CAD build for the part. Positions are in the model's coordinates, mm. Give positions to 0.01 mm unless a question says otherwise; leave off trailing zeros. Order: outer loops, then holes, each group sorted by start corner. A loop starts at its lowest first (then second) coordinate and runs counter-clockwise, first axis right, second up. Notation, with made-up numbers: (-38.75, 18.5) -> (-18.75, 18.5) arc R24 ccw to (-18.75, 49.5) -> close; hole circle Ø1 at (0.5, 57). An arc over 180 degrees is marked (long way). Answer as CSV lines item,"result".
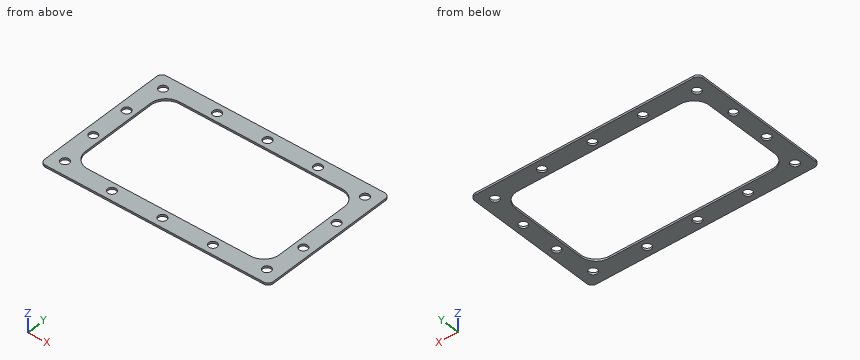
```python
from build123d import *

# Parameters (mm, degrees)
SKETCH1_W           = 112
SKETCH1_H           = 70
BOSS_EXTRUDE1_DEPTH = 1
FILLET1_R           = 3
SKETCH3_W           = 94
SKETCH3_H           = 52
CUT_EXTRUDE2_DEPTH  = 67.045438904
FILLET2_R           = 7.5
CUT_EXTRUDE3_REACH  = 68.045
SKETCH4_R           = 1.6
SKETCH5_R           = 2.05
CUT_EXTRUDE4_DEPTH  = 67.045438904
SKETCH6_W           = 132
SKETCH6_H           = 90
CUT_EXTRUDE5_DEPTH  = 67.045438904


with BuildPart() as part:
    # Sketch1 → Boss-Extrude1 (new body)
    with BuildSketch(Plane.XY):
        Rectangle(SKETCH1_W, SKETCH1_H)
    extrude(amount=BOSS_EXTRUDE1_DEPTH)

    # Fillet1
    fillet1_edges = [part.edges().sort_by_distance(p)[0] for p in [
        (-56, 35, 0.5),
        (56, 35, 0.5),
        (56, -35, 0.5),
        (-56, -35, 0.5),
    ]]
    fillet(fillet1_edges, radius=FILLET1_R)

    # Sketch3 → Cut-Extrude2 (cut, through all)
    with BuildSketch(Plane(origin=(0, 0, 0), x_dir=(-1, 0, 0), z_dir=(0, 0, -1))):
        Rectangle(SKETCH3_W, SKETCH3_H)
    extrude(amount=-CUT_EXTRUDE2_DEPTH, mode=Mode.SUBTRACT)

    # Fillet2
    fillet2_edges = [part.edges().sort_by_distance(p)[0] for p in [
        (-47, 26, 0.5),
        (-47, -26, 0.5),
        (47, -26, 0.5),
        (47, 26, 0.5),
    ]]
    fillet(fillet2_edges, radius=FILLET2_R)

    # Sketch4 → Cut-Extrude3 (cut, up to next)
    with BuildSketch(Plane(origin=(0, 0, 0), x_dir=(-1, 0, 0), z_dir=(0, 0, -1)), mode=Mode.PRIVATE) as cut_extrude3_sk1:
        with Locations((49, -28)):
            Circle(SKETCH4_R)
    cut_extrude3_tool1 = extrude(cut_extrude3_sk1.sketch, amount=-CUT_EXTRUDE3_REACH, mode=Mode.PRIVATE) & part.part
    # Sketch4 → Cut-Extrude3 (cut, up to next)
    with BuildSketch(Plane(origin=(0, 0, 0), x_dir=(-1, 0, 0), z_dir=(0, 0, -1)), mode=Mode.PRIVATE) as cut_extrude3_sk2:
        with Locations((24.5, -30)):
            Circle(SKETCH4_R)
    cut_extrude3_tool2 = extrude(cut_extrude3_sk2.sketch, amount=-CUT_EXTRUDE3_REACH, mode=Mode.PRIVATE) & part.part
    # Sketch4 → Cut-Extrude3 (cut, up to next)
    with BuildSketch(Plane(origin=(0, 0, 0), x_dir=(-1, 0, 0), z_dir=(0, 0, -1)), mode=Mode.PRIVATE) as cut_extrude3_sk3:
        with Locations((0, -30)):
            Circle(SKETCH4_R)
    cut_extrude3_tool3 = extrude(cut_extrude3_sk3.sketch, amount=-CUT_EXTRUDE3_REACH, mode=Mode.PRIVATE) & part.part
    # Sketch4 → Cut-Extrude3 (cut, up to next)
    with BuildSketch(Plane(origin=(0, 0, 0), x_dir=(-1, 0, 0), z_dir=(0, 0, -1)), mode=Mode.PRIVATE) as cut_extrude3_sk4:
        with Locations((-24.5, -30)):
            Circle(SKETCH4_R)
    cut_extrude3_tool4 = extrude(cut_extrude3_sk4.sketch, amount=-CUT_EXTRUDE3_REACH, mode=Mode.PRIVATE) & part.part
    # Sketch4 → Cut-Extrude3 (cut, up to next)
    with BuildSketch(Plane(origin=(0, 0, 0), x_dir=(-1, 0, 0), z_dir=(0, 0, -1)), mode=Mode.PRIVATE) as cut_extrude3_sk5:
        with Locations((-49, -28)):
            Circle(SKETCH4_R)
    cut_extrude3_tool5 = extrude(cut_extrude3_sk5.sketch, amount=-CUT_EXTRUDE3_REACH, mode=Mode.PRIVATE) & part.part
    # Sketch4 → Cut-Extrude3 (cut, up to next)
    with BuildSketch(Plane(origin=(0, 0, 0), x_dir=(-1, 0, 0), z_dir=(0, 0, -1)), mode=Mode.PRIVATE) as cut_extrude3_sk6:
        with Locations((-51, -9.5)):
            Circle(SKETCH4_R)
    cut_extrude3_tool6 = extrude(cut_extrude3_sk6.sketch, amount=-CUT_EXTRUDE3_REACH, mode=Mode.PRIVATE) & part.part
    # Sketch4 → Cut-Extrude3 (cut, up to next)
    with BuildSketch(Plane(origin=(0, 0, 0), x_dir=(-1, 0, 0), z_dir=(0, 0, -1)), mode=Mode.PRIVATE) as cut_extrude3_sk7:
        with Locations((-51, 9.5)):
            Circle(SKETCH4_R)
    cut_extrude3_tool7 = extrude(cut_extrude3_sk7.sketch, amount=-CUT_EXTRUDE3_REACH, mode=Mode.PRIVATE) & part.part
    # Sketch4 → Cut-Extrude3 (cut, up to next)
    with BuildSketch(Plane(origin=(0, 0, 0), x_dir=(-1, 0, 0), z_dir=(0, 0, -1)), mode=Mode.PRIVATE) as cut_extrude3_sk8:
        with Locations((-49, 28)):
            Circle(SKETCH4_R)
    cut_extrude3_tool8 = extrude(cut_extrude3_sk8.sketch, amount=-CUT_EXTRUDE3_REACH, mode=Mode.PRIVATE) & part.part
    # Sketch4 → Cut-Extrude3 (cut, up to next)
    with BuildSketch(Plane(origin=(0, 0, 0), x_dir=(-1, 0, 0), z_dir=(0, 0, -1)), mode=Mode.PRIVATE) as cut_extrude3_sk9:
        with Locations((-24.5, 30)):
            Circle(SKETCH4_R)
    cut_extrude3_tool9 = extrude(cut_extrude3_sk9.sketch, amount=-CUT_EXTRUDE3_REACH, mode=Mode.PRIVATE) & part.part
    # Sketch4 → Cut-Extrude3 (cut, up to next)
    with BuildSketch(Plane(origin=(0, 0, 0), x_dir=(-1, 0, 0), z_dir=(0, 0, -1)), mode=Mode.PRIVATE) as cut_extrude3_sk10:
        with Locations((0, 30)):
            Circle(SKETCH4_R)
    cut_extrude3_tool10 = extrude(cut_extrude3_sk10.sketch, amount=-CUT_EXTRUDE3_REACH, mode=Mode.PRIVATE) & part.part
    # Sketch4 → Cut-Extrude3 (cut, up to next)
    with BuildSketch(Plane(origin=(0, 0, 0), x_dir=(-1, 0, 0), z_dir=(0, 0, -1)), mode=Mode.PRIVATE) as cut_extrude3_sk11:
        with Locations((24.5, 30)):
            Circle(SKETCH4_R)
    cut_extrude3_tool11 = extrude(cut_extrude3_sk11.sketch, amount=-CUT_EXTRUDE3_REACH, mode=Mode.PRIVATE) & part.part
    # Sketch4 → Cut-Extrude3 (cut, up to next)
    with BuildSketch(Plane(origin=(0, 0, 0), x_dir=(-1, 0, 0), z_dir=(0, 0, -1)), mode=Mode.PRIVATE) as cut_extrude3_sk12:
        with Locations((49, 28)):
            Circle(SKETCH4_R)
    cut_extrude3_tool12 = extrude(cut_extrude3_sk12.sketch, amount=-CUT_EXTRUDE3_REACH, mode=Mode.PRIVATE) & part.part
    # Sketch4 → Cut-Extrude3 (cut, up to next)
    with BuildSketch(Plane(origin=(0, 0, 0), x_dir=(-1, 0, 0), z_dir=(0, 0, -1)), mode=Mode.PRIVATE) as cut_extrude3_sk13:
        with Locations((51, 9.5)):
            Circle(SKETCH4_R)
    cut_extrude3_tool13 = extrude(cut_extrude3_sk13.sketch, amount=-CUT_EXTRUDE3_REACH, mode=Mode.PRIVATE) & part.part
    # Sketch4 → Cut-Extrude3 (cut, up to next)
    with BuildSketch(Plane(origin=(0, 0, 0), x_dir=(-1, 0, 0), z_dir=(0, 0, -1)), mode=Mode.PRIVATE) as cut_extrude3_sk14:
        with Locations((51, -9.5)):
            Circle(SKETCH4_R)
    cut_extrude3_tool14 = extrude(cut_extrude3_sk14.sketch, amount=-CUT_EXTRUDE3_REACH, mode=Mode.PRIVATE) & part.part
    add(cut_extrude3_tool1.solids().sort_by_distance((-49, -28, 0))[0], mode=Mode.SUBTRACT)
    add(cut_extrude3_tool2.solids().sort_by_distance((-24.5, -30, 0))[0], mode=Mode.SUBTRACT)
    add(cut_extrude3_tool3.solids().sort_by_distance((0, -30, 0))[0], mode=Mode.SUBTRACT)
    add(cut_extrude3_tool4.solids().sort_by_distance((24.5, -30, 0))[0], mode=Mode.SUBTRACT)
    add(cut_extrude3_tool5.solids().sort_by_distance((49, -28, 0))[0], mode=Mode.SUBTRACT)
    add(cut_extrude3_tool6.solids().sort_by_distance((51, -9.5, 0))[0], mode=Mode.SUBTRACT)
    add(cut_extrude3_tool7.solids().sort_by_distance((51, 9.5, 0))[0], mode=Mode.SUBTRACT)
    add(cut_extrude3_tool8.solids().sort_by_distance((49, 28, 0))[0], mode=Mode.SUBTRACT)
    add(cut_extrude3_tool9.solids().sort_by_distance((24.5, 30, 0))[0], mode=Mode.SUBTRACT)
    add(cut_extrude3_tool10.solids().sort_by_distance((0, 30, 0))[0], mode=Mode.SUBTRACT)
    add(cut_extrude3_tool11.solids().sort_by_distance((-24.5, 30, 0))[0], mode=Mode.SUBTRACT)
    add(cut_extrude3_tool12.solids().sort_by_distance((-49, 28, 0))[0], mode=Mode.SUBTRACT)
    add(cut_extrude3_tool13.solids().sort_by_distance((-51, 9.5, 0))[0], mode=Mode.SUBTRACT)
    add(cut_extrude3_tool14.solids().sort_by_distance((-51, -9.5, 0))[0], mode=Mode.SUBTRACT)

    # Sketch5 → Cut-Extrude4 (cut, through all)
    with BuildSketch(Plane.XY.offset(1)):
        with Locations((-49, 28)):
            Circle(SKETCH5_R)
        with Locations((-24.5, 30)):
            Circle(SKETCH5_R)
        with Locations((0, 30)):
            Circle(SKETCH5_R)
        with Locations((24.5, 30)):
            Circle(SKETCH5_R)
        with Locations((49, 28)):
            Circle(SKETCH5_R)
        with Locations((51, 9.5)):
            Circle(SKETCH5_R)
        with Locations((51, -9.5)):
            Circle(SKETCH5_R)
        with Locations((49, -28)):
            Circle(SKETCH5_R)
        with Locations((24.5, -30)):
            Circle(SKETCH5_R)
        with Locations((0, -30)):
            Circle(SKETCH5_R)
        with Locations((-24.5, -30)):
            Circle(SKETCH5_R)
        with Locations((-49, -28)):
            Circle(SKETCH5_R)
        with Locations((-51, -9.5)):
            Circle(SKETCH5_R)
        with Locations((-51, 9.5)):
            Circle(SKETCH5_R)
    extrude(amount=-CUT_EXTRUDE4_DEPTH, mode=Mode.SUBTRACT)

    # Sketch6 → Cut-Extrude5 (cut, through all)
    with BuildSketch(Plane.XY.offset(1)):
        Rectangle(SKETCH6_W, SKETCH6_H)
        with BuildLine():
            Line((-53, 34.5), (53, 34.5))
            ThreePointArc((53, 34.5), (54.767766953, 33.767766953), (55.5, 32))
            Line((55.5, 32), (55.5, -32))
            ThreePointArc((55.5, -32), (54.767766953, -33.767766953), (53, -34.5))
            Line((53, -34.5), (-53, -34.5))
            ThreePointArc((-53, -34.5), (-54.767766953, -33.767766953), (-55.5, -32))
            Line((-55.5, -32), (-55.5, 32))
            ThreePointArc((-55.5, 32), (-54.767766953, 33.767766953), (-53, 34.5))
        make_face(mode=Mode.SUBTRACT)
    extrude(amount=-CUT_EXTRUDE5_DEPTH, mode=Mode.SUBTRACT)


solid = part.part
```
1) Wall check: line 1 along Y through (x, z) = (-24.5, 0.4); line 2 along Y through (x, z) = (40.5, 0.15); line 3 along Y through (x, z) = (7.5, 0.3). Give the ranges that are in metal, low to high. Write a range as [from, to].
Data:
line 1,"y = [-34.5, -32.05], [-27.95, -26], [26, 27.95], [32.05, 34.5]"
line 2,"y = [-34.5, -25.93], [25.93, 34.5]"
line 3,"y = [-34.5, -26], [26, 34.5]"
2) Band-saw the part on B-B, the plane z = 0.15. Give the number of separate pieces and of enclosed holes in the cut face, then the cut area to 3 significant figures.
Data:
separate pieces,"1"
enclosed holes,"15"
area,"2,630 mm2"
3) Band-saw the part on C-C, the plane y = 6. Write the cut outline in (x, z).
Data:
outline,"(-55.5, 0) -> (-47, 0) -> (-47, 1) -> (-55.5, 1) -> close; (47, 0) -> (55.5, 0) -> (55.5, 1) -> (47, 1) -> close"
4) Band-saw the part on D-D, the plane x = -24. Write the cut outline in (y, z), then the cut area to 3 significant figures.
Data:
outline,"(-34.5, 0) -> (-31.99, 0) -> (-31.99, 1) -> (-34.5, 1) -> close; (-28.01, 0) -> (-26, 0) -> (-26, 1) -> (-28.01, 1) -> close; (26, 0) -> (28.01, 0) -> (28.01, 1) -> (26, 1) -> close; (31.99, 0) -> (34.5, 0) -> (34.5, 1) -> (31.99, 1) -> close"
area,"9.05 mm2"
5) Band-saw the part on A-A, the plane x = 0. Write the cut outline in (y, z), then the cut area to 3 significant figures.
Data:
outline,"(-34.5, 0) -> (-32.05, 0) -> (-32.05, 1) -> (-34.5, 1) -> close; (-27.95, 0) -> (-26, 0) -> (-26, 1) -> (-27.95, 1) -> close; (26, 0) -> (27.95, 0) -> (27.95, 1) -> (26, 1) -> close; (32.05, 0) -> (34.5, 0) -> (34.5, 1) -> (32.05, 1) -> close"
area,"8.80 mm2"
